Here's the drawing with two shaded views (mm, measured from the low corner). I have some questions. A direction names the side the tool comes from. Give positions to 0.01 mm unless a question says otherwise; leave off trailing zeros. Loops run counter-clockwise (first coordinate to the right, second up) from the corner with the lowest first, then second, coordinate; pieces in that order, holes last. Notation, with made-up numbers: (0.25, 43.5) - (42.25, 43.5) arc R9 ccw to (42.25, 48.5) - close; hole circle Ø3 at (22, -32.75). An arc over 180 degrees is marked (long way). Use a Markdown table: item, result. Add a question column.
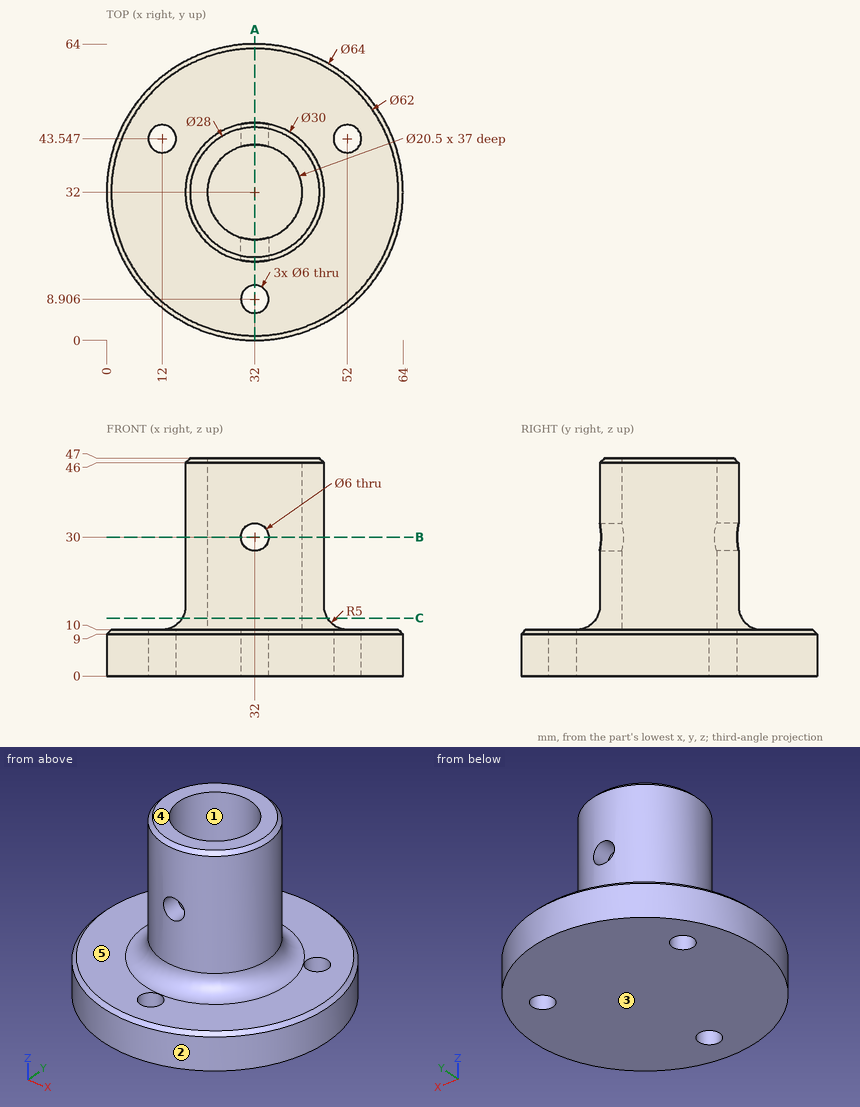
1. Suppose I cut it at A-A (x = 32). State how many separate pieces and enclosed holes the cut face has, and give its area (3 significant figures).
2. Suppose I cut it at B-B (z = 30). List the corners of the cut face in (x, y) for me.
3. If we mould it in two halves opening along X, with no side actions, what happens to the marked faces 1, 2 and 3? For each: released by +X, released by -X, zero draft, split by the parting line, or undercut.
4. Suppose I cut it at C-C (z = 12.5). List the corners of the cut face in (x, y) for me, and give its area (3 significant figures).
5. Will these pins go through, and if not, where does the flat tip stop? P1, Ø8, axis at x = 52, y = 43.55, coming from the +Z side; P2, Ø4, axis at x = 42, z = 18.5, coming from the -Y side; P3, Ø12, axis at x = 23, z = 26, coming from the -Y side.
6. On a 3-axis mill with a long thin cutter (end or side, diameter ignored), from which of +Z, -Z, +X, -X, +Y, -Y can I reach the whole of each face in a straight line? I mean the marked faces 4 and 5. Say none if no direction works.
7. Please list where these lines run through material, in increasing order: line 1 along Y through (x, z) = (32, 2.25); line 2 along Z through (x, y) = (32, 44.95); line 3 along X through (y, z) = (37.5, 27.5). Write a range as [from, to].
Results below:
| question | item | result |
|---|---|---|
| 1 | separate pieces | 4 |
| 1 | enclosed holes | 0 |
| 1 | area | 883 mm² |
| 2 | outline | (29, 17.3) - (29, 22.2) arc R10.25 cw to (29, 41.8) - (29, 46.7) arc R15 ccw to start; (35, 17.3) arc R15 ccw to (35, 46.7) - (35, 41.8) arc R10.25 cw to (35, 22.2) - close |
| 3 | face 1 | undercut |
| 3 | face 2 | split by the parting line |
| 3 | face 3 | zero draft |
| 4 | outline | circle Ø31.34 at (32, 32); hole circle Ø20.5 at (32, 32) |
| 4 | area | 441 mm² |
| 5 | P1 | z = 10.08 |
| 5 | P2 | y = 19.31 |
| 5 | P3 | y = 17.3 |
| 6 | face 4 | +Z, +X, -X, +Y, -Y |
| 6 | face 5 | +Z |
| 7 | line 1 | [0, 5.91], [11.91, 64] |
| 7 | line 2 | [0, 27], [33, 47] |
| 7 | line 3 | [18.04, 23.35], [40.65, 45.96] |
